Check sheet for the modelled part. Datum: model origin and axes. Units: mm. A direction names the side the tool comes from. Round coordinates to 2 decimals unless told otherwise and drop trailing zeros. Write each loop counter-clockwise with the first axis right and the second up, starting at its lowest first coordinate (ties: lowest second). Pieces come first, ordered by that corner, then holes. Notation, with made-up numbers: (65.25, -29.75) -> (79.25, -29.75) arc R35 cw to (79.25, 8.25) -> close; hole circle Ø10 at (3, -1.75). An arc over 180 degrees is marked (long way). Write item = value, one per line.
from build123d import *

# Parameters (mm, degrees)
SKETCH1_W           = 76.2
SKETCH1_H           = 76.2
BOSS_EXTRUDE1_DEPTH = 38.1
SKETCH3_W           = 39.463440316
SKETCH3_H           = 70.199999808
SKETCH3_W_2         = 39.34827811
CUT_EXTRUDE1_DEPTH  = 35.100000006
SKETCH4_R           = 3.937
CUT_EXTRUDE2_DEPTH  = 38.1


with BuildPart() as part:
    # Sketch1 → Boss-Extrude1 (new body)
    with BuildSketch(Plane.XY):
        Rectangle(SKETCH1_W, SKETCH1_H)
    extrude(amount=BOSS_EXTRUDE1_DEPTH)

    # Sketch3 → Cut-Extrude1 (cut)
    with BuildSketch(Plane.XY.offset(38.1)):
        with Locations((21.231720251, 0)):
            Rectangle(SKETCH3_W, SKETCH3_H)
        with Locations((-21.174138956, 0)):
            Rectangle(SKETCH3_W_2, SKETCH3_H)
    extrude(amount=-CUT_EXTRUDE1_DEPTH, mode=Mode.SUBTRACT)

    # Sketch4 → Cut-Extrude2 (cut, symmetric)
    with BuildSketch(Plane(origin=(0, 0, 0), x_dir=(1, 0, 0), z_dir=(0, 1, 0))):
        with Locations(Location((19.05, -19.05, 0), (0, 0, 270))):
            Circle(SKETCH4_R)
        with Locations(Location((-19.05, -19.05, 0), (0, 0, 270))):
            Circle(SKETCH4_R)
    extrude(amount=CUT_EXTRUDE2_DEPTH, both=True, mode=Mode.SUBTRACT)


solid = part.part
(1) Release check for a two-part mould opening along Y. For faces 1 (the flat face through (20, -35.1, 25)), 2 (the cylindrical face through (-15.147, 36.621, 18.537)), 3 (the flat face through (-20, 0, 3)), 4 (the flat face through (-1, 38.1, 19)) record: pulls with the +Y half, pulls with the -Y half, needs draft (parallel to the pull), parting line crosses it, or undercut.
Worked answers:
face_1 = undercut
face_2 = needs draft
face_3 = undercut
face_4 = pulls with the +Y half
(2) Sectioned sample at B-B on y = -15. Enter the section's corners in (x, z).
Worked answers:
outline = (-38.1, 0) -> (38.1, 0) -> (38.1, 3) -> (1.5, 3) -> (1.5, 38.1) -> (-1.5, 38.1) -> (-1.5, 3) -> (-38.1, 3) -> close
(3) Go/stop test with flat-tipped pins: P1, Ø12, axis at x = -21, y = 12, coming from the +Z side; P2, Ø10.5, axis at y = -14.5, z = 14.5, coming from the +X side; P3, Ø6, axis at x = 21.5, y = 15, coming from the -Z side; P4, Ø2, axis at y = -2.5, z = 30, coming from the -X side. Record where each tip stops, or that it passes through.
Worked answers:
P1 = 3
P2 = 1.5
P3 = 0
P4 = -1.5
(4) Sectioned sample at C-C on x = -19.05. Enter the section's corners in (y, z), then the cut area to 3 significant figures.
Worked answers:
outline = (-38.1, 0) -> (38.1, 0) -> (38.1, 15.11) -> (35.1, 15.11) -> (35.1, 3) -> (-35.1, 3) -> (-35.1, 15.11) -> (-38.1, 15.11) -> close; (-38.1, 22.99) -> (-35.1, 22.99) -> (-35.1, 38.1) -> (-38.1, 38.1) -> close; (35.1, 22.99) -> (38.1, 22.99) -> (38.1, 38.1) -> (35.1, 38.1) -> close
area = 392 mm²
(5) Sectioned sample at D-D on x = 4.5. Enter the section's corners in (y, z).
Worked answers:
outline = (-38.1, 0) -> (38.1, 0) -> (38.1, 38.1) -> (35.1, 38.1) -> (35.1, 3) -> (-35.1, 3) -> (-35.1, 38.1) -> (-38.1, 38.1) -> close
(6) Access from +Z, -Z, +X, -X, +Y, -Y to the whole of each face (thin tool, end or side, straight path). Record for faces 5 (the flat face through (38.1, -3, 2)), 6 (the flat face through (1.5, 0, 21)), 7 (the flat face through (-1.5, 0, 21)).
Worked answers:
face_5 = +Z, -Z, +X, +Y, -Y
face_6 = +Z, +X
face_7 = +Z, -X
(7) Material ranges on L1, parallel to X at y = -37.3, z = 19.05; L2, parallel to Y at x = 33.5, z = 8; L3, parallel to X at y = -1, z = 24, recorded low to high. Write a range as [from, to].
Worked answers:
L1 = [-38.1, -22.99], [-15.11, 15.11], [22.99, 38.1]
L2 = [-38.1, -35.1], [35.1, 38.1]
L3 = [-1.5, 1.5]
(8) Sectioned sample at A-A on z = 19.05. Enter the section's corners in (x, y), then the cut area to 3 significant figures.
Worked answers:
outline = (-38.1, -38.1) -> (-22.99, -38.1) -> (-22.99, -35.1) -> (-38.1, -35.1) -> close; (-38.1, 35.1) -> (-22.99, 35.1) -> (-22.99, 38.1) -> (-38.1, 38.1) -> close; (-15.11, -38.1) -> (15.11, -38.1) -> (15.11, -35.1) -> (1.5, -35.1) -> (1.5, 35.1) -> (15.11, 35.1) -> (15.11, 38.1) -> (-15.11, 38.1) -> (-15.11, 35.1) -> (-1.5, 35.1) -> (-1.5, -35.1) -> (-15.11, -35.1) -> close; (22.99, -38.1) -> (38.1, -38.1) -> (38.1, -35.1) -> (22.99, -35.1) -> close; (22.99, 35.1) -> (38.1, 35.1) -> (38.1, 38.1) -> (22.99, 38.1) -> close
area = 573 mm²
